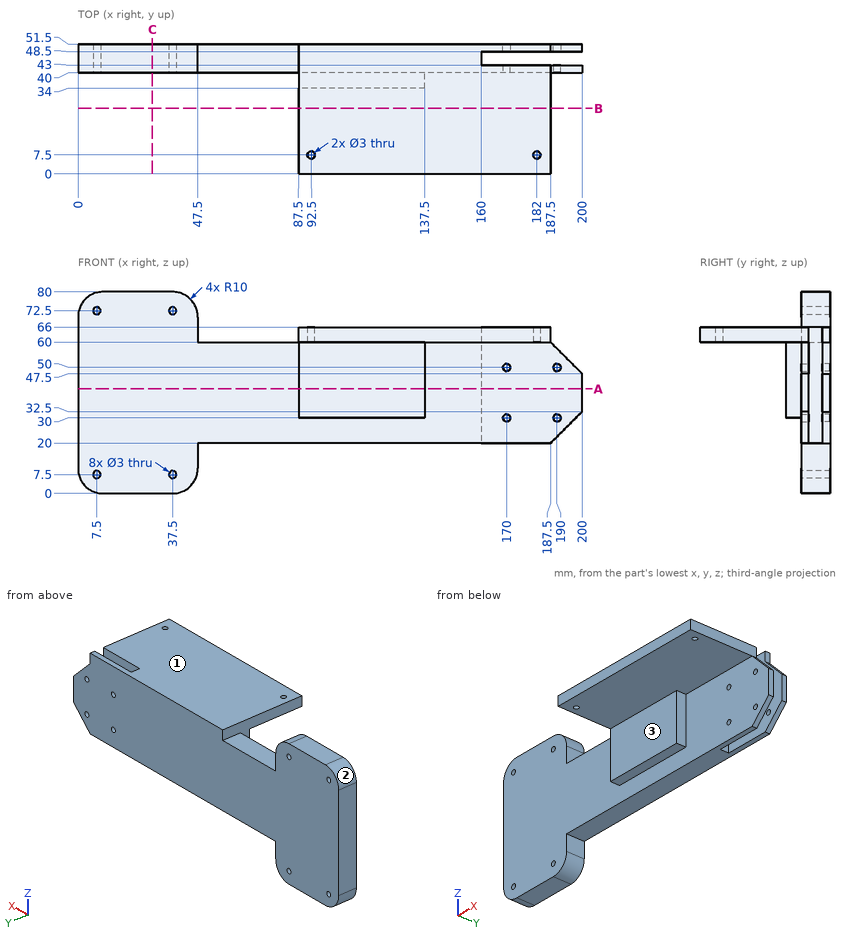
Geometry: see drawing. Coordinates: mm, zero at the bounding-box minimum. A direction names the side the tool comes from. Round coordinates to 2 decimals unless told otherwise and drop trailing zeros. Write each loop counter-clockwise with the first axis right and the second up, starting at its lowest first coordinate (ties: lowest second). Pieces come first, ordered by that corner, then holes.
Item 1: Section query C-C (x = 29.5). Return loops of the section in (y, z).
Item 2: Section query A-A (z = 41.5). Return loops of the section in (x, y), plus the area to 3 significant figures.
Item 3: Set-up query: the marked faces 1, 2 and 3. Return all of +Z, -Z, +X, -X, +Y, -Y with unobstructed straight access to the full face (end or side cutting, diameter ignored); none if empty.
Item 4: Material intervals for L1, parallel to Z at x = 170, y = 42.3; L2, parallel to Y at x = 160.5, z = 21; L3, parallel to X at y = 42, z = 30, sorted ascending.
Item 5: Pin query (flat end, axial travel): P1, Ø3, axis at y = 45, z = 54, coming from the +X side; P2, Ø1.5, axis at x = 86, z = 37, coming from the -Y side; P3, Ø6, axis at x = 64.5, y = 44.5, coming from the +Z side. Return the tip coordinate at first contact, or that it passes through.
Item 6: Section query B-B (y = 26). Return loops of the section in (x, z).
Completed:
1. outline: (40, 0) - (51.5, 0) - (51.5, 80) - (40, 80) - close
2. outline: (0, 40) - (87.5, 40) - (87.5, 34) - (137.5, 34) - (137.5, 40) - (200, 40) - (200, 43) - (160, 43) - (160, 48.5) - (200, 48.5) - (200, 51.5) - (0, 51.5) - close
2. area: 2,380 mm2
3. face 1: +Z, +X, +Y, -Y
3. face 2: +Z, -X, +Y, -Y
3. face 3: -Z, +X, -X, -Y
4. L1: z = 20 to 28.5, 31.5 to 48.5, 51.5 to 66
4. L2: y = 40 to 43, 48.5 to 51.5
4. L3: x = 0 to 168.5, 171.5 to 188.5, 191.5 to 197.5
5. P1: stops at x = 160
5. P2: stops at y = 40
5. P3: stops at z = 60
6. outline: (87.5, 60) - (187.5, 60) - (187.5, 66) - (87.5, 66) - close
